Build history of the part. All positions in model axes, mm. A direction names the side the tool comes from. Round coordinates to 2 decimals unless told otherwise and drop trailing zeros. Write each loop counter-clockwise with the first axis right and the second up, starting at its lowest first coordinate (ties: lowest second). Pieces come first, ordered by that corner, then holes. Notation, with made-up numbers: (-3.75, -16.75) -> (14.25, -16.75) arc R17 cw to (14.25, 16.25) -> close; hole circle Ø1 at (-27.5, 29). An arc over 180 degrees is marked (long way). One line per question, with ' | ' between items.
from build123d import *

# Parameters (mm, degrees)
SKETCH_R           = 70
SKETCH_R_2         = 2.5
PAD_DEPTH          = 12
SKETCH001_R        = 1.5
POCKET_DEPTH       = 15
SKETCH002_R        = 4
SKETCH002_R_2      = 1.5
PAD001_DEPTH       = 3.5
SKETCH003_R        = 2.5
POCKET001_DEPTH    = 15
POCKET002_DEPTH    = 5
POLARPATTERN_COUNT = 2


with BuildPart() as part:
    # Sketch → Pad (new body)
    with BuildSketch(Plane.XY):
        Circle(SKETCH_R)
        with Locations((38.6, 51.05)):
            Circle(SKETCH_R_2, mode=Mode.SUBTRACT)
        with Locations((-38.6, 51.05)):
            Circle(SKETCH_R_2, mode=Mode.SUBTRACT)
        with Locations((38.6, -51.05)):
            Circle(SKETCH_R_2, mode=Mode.SUBTRACT)
        with Locations((-38.6, -51.05)):
            Circle(SKETCH_R_2, mode=Mode.SUBTRACT)
    extrude(amount=PAD_DEPTH)

    # Sketch001 (on Face7 of Pad) → Pocket (cut)
    with BuildSketch(Plane.XY.offset(12)):
        with Locations((-31, 41)):
            Circle(SKETCH001_R)
        with Locations((31, 41)):
            Circle(SKETCH001_R)
        with Locations((31, -41)):
            Circle(SKETCH001_R)
        with Locations((-31, -41)):
            Circle(SKETCH001_R)
    extrude(amount=-POCKET_DEPTH, mode=Mode.SUBTRACT)

    # Sketch002 (on Face3 of Pocket) → Pad001 (join)
    with BuildSketch(Plane.XY.offset(12)):
        with Locations((-31, -41)):
            Circle(SKETCH002_R)
        with Locations((-31, -41)):
            Circle(SKETCH002_R_2, mode=Mode.SUBTRACT)
        with Locations((31, -41)):
            Circle(SKETCH002_R)
        with Locations((31, -41)):
            Circle(SKETCH002_R_2, mode=Mode.SUBTRACT)
        with Locations((31, 41)):
            Circle(SKETCH002_R)
        with Locations((31, 41)):
            Circle(SKETCH002_R_2, mode=Mode.SUBTRACT)
        with Locations((-31, 41)):
            Circle(SKETCH002_R)
        with Locations((-31, 41)):
            Circle(SKETCH002_R_2, mode=Mode.SUBTRACT)
    extrude(amount=PAD001_DEPTH)

    # Sketch003 (on Face3 of Pad001) → Pocket001 (cut)
    with BuildSketch(Plane.XY.offset(12)):
        with Locations((0, 58)):
            Circle(SKETCH003_R)
        with Locations((50.229473, 29)):
            Circle(SKETCH003_R)
        with Locations((50.229473, -29)):
            Circle(SKETCH003_R)
        with Locations((0, -58)):
            Circle(SKETCH003_R)
        with Locations((-50.229473, 29)):
            Circle(SKETCH003_R)
    extrude(amount=-POCKET001_DEPTH, mode=Mode.SUBTRACT)

    # Sketch004 (on Face2 of Pocket001) → Pocket002 (cut)
    with BuildSketch(Plane(origin=(0, 0, 0), x_dir=(1, 0, 0), z_dir=(0, 0, -1))):
        Polygon((-35.008085, 53.766274), (-39.156405, 55.518827), (-42.74832, 52.802553), (-42.191915, 48.333726), (-38.043595, 46.581173), (-34.45168, 49.297447), align=None)
        Polygon((-28.513289, 42.880497), (-31.385203, 44.093803), (-33.871914, 42.213306), (-33.486711, 39.119503), (-30.614797, 37.906197), (-28.128086, 39.786694), align=None)
        Polygon((-35.008085, -53.766274), (-34.45168, -49.297447), (-38.043595, -46.581173), (-42.191915, -48.333726), (-42.74832, -52.802553), (-39.156405, -55.518827), align=None)
        Polygon((-28.513289, -42.880497), (-28.128086, -39.786694), (-30.614797, -37.906197), (-33.486711, -39.119503), (-33.871914, -42.213306), (-31.385203, -44.093803), align=None)
    pocket002 = extrude(amount=-POCKET002_DEPTH, mode=Mode.SUBTRACT)

    # PolarPattern: Pocket002 ×2 about axis
    polarpattern_axis = Axis((0, 0, 0), (0, 0, -1))
    for i in range(1, POLARPATTERN_COUNT):
        add(pocket002.rotate(polarpattern_axis, i * 360 / POLARPATTERN_COUNT), mode=Mode.SUBTRACT)


solid = part.part
(1) Slice it at B-B (y = 51.05). Write the cut outline in (x, z), then the cut area to 3 significant figures.
Calculated:
outline: (-47.89, 0) -> (-42.53, 0) -> (-42.53, 5) -> (-41.1, 5) -> (-41.1, 12) -> (-47.89, 12) -> close; (-36.1, 5) -> (-34.67, 5) -> (-34.67, 0) -> (34.67, 0) -> (34.67, 5) -> (36.1, 5) -> (36.1, 12) -> (-36.1, 12) -> close; (41.1, 5) -> (42.53, 5) -> (42.53, 0) -> (47.89, 0) -> (47.89, 12) -> (41.1, 12) -> close | area: 1,000 mm2
(2) 3-axis set-ups, long thin cutter, end or side, ignore diameter. For faces 1 (the cylindrical face through (36.76, -49.36, 8.45)), 2 (the flat face through (-28.323, 41.355, 2.465)), 3 (the cylindrical face through (30.479, -37.034, 13.726)): which of +Z, -Z, +X, -X, +Y, -Y reach the whole face in a straight line?
Calculated:
face 1: +Z, -Z | face 2: -Z | face 3: +Z
(3) Drop flat-ended pins along their axis: pin 1 (5 mm diameter, centred on y = 17, z = 11.5, fed in from +X); pin 2 (4 mm diameter, centred on x = 31, y = -41, fed in from -Z); pin 3 (1.5 mm diameter, centred on x = 36, y = 13, fed in from +Z); pin 4 (4 mm diameter, centred on x = 0, y = -58, fed in from -Z). Give the stop position or say it passes through.
Calculated:
pin 1: x = 68.48 | pin 2: z = 5 | pin 3: z = 12 | pin 4: through
(4) Slice it at C-C (y = -58). Write the cut outline in (x, z), then the cut area to 3 significant figures.
Calculated:
outline: (-39.19, 0) -> (-2.5, 0) -> (-2.5, 12) -> (-39.19, 12) -> close; (2.5, 0) -> (39.19, 0) -> (39.19, 12) -> (2.5, 12) -> close | area: 881 mm2
(5) Slice it at A-A (z = 9.25). State how many separate pieces and enclosed holes the cut face has, then the cut area to 3 significant figures.
Calculated:
separate pieces: 1 | enclosed holes: 13 | area: 15,200 mm2
(6) Slice it at D-D (x = 23.5). Write the cut outline in (y, z), then the cut area to 3 significant figures.
Calculated:
outline: (-65.94, 0) -> (65.94, 0) -> (65.94, 12) -> (-65.94, 12) -> close | area: 1,580 mm2
(7) Wall check: line 1 (Y direction, x = 0, z = 3.5); line 2 (Y direction, x = 1, z = 10.5); line 3 (X direction, y = -51.05, z = 8.5). Give the ranges that are in metal, low to high. Write a range as from..to.
Calculated:
line 1: -70..-60.5, -55.5..55.5, 60.5..70 | line 2: -69.99..-60.29, -55.71..55.71, 60.29..69.99 | line 3: -47.89..-41.1, -36.1..36.1, 41.1..47.89
